```python
from build123d import *

# Parameters (mm, degrees)
SKETCH4_W                        = 24.1
SKETCH4_H                        = 23.8
BOSS_EXTRUDE2_DEPTH              = 2
SKETCH1_W                        = 28.1
SKETCH1_H                        = 28.7
SKETCH1_W_2                      = 24.1
SKETCH1_H_2                      = 23.8
BOSS_EXTRUDE3_DEPTH              = 4
SKETCH6_W                        = 2
SKETCH6_H                        = 2.5
CUT_EXTRUDE2_DEPTH               = 2
SKETCH8_W                        = 7
SKETCH8_H                        = 2
BOSS_EXTRUDE4_DEPTH              = 11.8
SKETCH11_R                       = 6
CUT_EXTRUDE4_DEPTH               = 4
SKETCH12_W                       = 10
SKETCH12_H                       = 2
BOSS_EXTRUDE5_DEPTH              = 7.9
FILLET9_R                        = 5
FILLET10_R                       = 5
SKETCH14_R                       = 2.3
BOSS_EXTRUDE6_DEPTH              = 2.5
DOME3_FACE_RADIUS                = 2.3
DOME3_HEIGHT                     = 1
FILLET11_R                       = 2
FILLET12_R                       = 2
FILLET13_R                       = 2
FILLET14_R                       = 2
BOSS_EXTRUDE7_DEPTH              = 3
SKETCH19_R                       = 0.3
CUT_EXTRUDE6_DEPTH               = 2
CBORE_START                      = -0.2
CBORE_FOR_M1_6_SHCS1_OUTLINE_R   = 1.85
CBORE_FOR_M1_6_SHCS1_DEPTH       = 2.2
CBORE_START_2                    = -3
CBORE_FOR_M1_6_SHCS1_2_OUTLINE_R = 1
CBORE_FOR_M1_6_SHCS1_2_DEPTH     = 2.8
CUT_EXTRUDE8_DEPTH               = 2


# Read off the part's stored shape, not the designer's step: CBORE for M1.6 SHCS1
with BuildPart() as part:
    # Sketch4 → Boss-Extrude2 (new body)
    with BuildSketch(Plane.XY):
        with Locations((14.05, 13.9)):
            Rectangle(SKETCH4_W, SKETCH4_H)
    extrude(amount=BOSS_EXTRUDE2_DEPTH)

    # Sketch1 → Boss-Extrude3 (add)
    with BuildSketch(Plane.XY):
        with Locations((14.05, 14.35)):
            Rectangle(SKETCH1_W, SKETCH1_H)
        with Locations((14.05, 13.9)):
            Rectangle(SKETCH1_W_2, SKETCH1_H_2, mode=Mode.SUBTRACT)
    extrude(amount=BOSS_EXTRUDE3_DEPTH)

    # Sketch6 → Cut-Extrude2 (cut)
    with BuildSketch(Plane.XY.offset(4)):
        with Locations((1, 19.15)):
            Rectangle(SKETCH6_W, SKETCH6_H)
        with Locations((27.1, 19.15)):
            Rectangle(SKETCH6_W, SKETCH6_H)
    extrude(amount=-CUT_EXTRUDE2_DEPTH, mode=Mode.SUBTRACT)

    # Sketch8 → Boss-Extrude4 (add)
    with BuildSketch(Plane.XY):
        with Locations((-1.5, 21.4)):
            Rectangle(SKETCH8_W, SKETCH8_H)
        with Locations((29.6, 21.4)):
            Rectangle(SKETCH8_W, SKETCH8_H)
    extrude(amount=BOSS_EXTRUDE4_DEPTH)

    # Sketch11 → Cut-Extrude4 (cut)
    with BuildSketch(Plane(origin=(0, 25.8, 0), x_dir=(-1, 0, 0), z_dir=(0, -1, 0))):
        with Locations((-8, -8)):
            Circle(SKETCH11_R)
    extrude(amount=-CUT_EXTRUDE4_DEPTH, mode=Mode.SUBTRACT)

    # Sketch12 → Boss-Extrude5 (add)
    with BuildSketch(Plane.XY.offset(4)):
        with Locations((7.9, 1)):
            Rectangle(SKETCH12_W, SKETCH12_H)
    extrude(amount=BOSS_EXTRUDE5_DEPTH)

    # Fillet9
    fillet9_edges = [part.edges().sort_by_distance(p)[0] for p in [
        (2.9, 1, 11.9),
    ]]
    fillet(fillet9_edges, radius=FILLET9_R)

    # Fillet10
    fillet10_edges = [part.edges().sort_by_distance(p)[0] for p in [
        (12.9, 1, 11.9),
    ]]
    fillet(fillet10_edges, radius=FILLET10_R - 0.0001)  # a hair under: the kernel refuses the full size

    # Sketch14 → Boss-Extrude6 (add)
    with BuildSketch(Plane(origin=(0, 0, 0), x_dir=(-1, 0, 0), z_dir=(0, -1, 0))):
        with Locations(Location((-7.9, -7.9, 0), (0, 0, 270))):
            Circle(SKETCH14_R)
    extrude(amount=BOSS_EXTRUDE6_DEPTH)

    # Dome3: a dome of height H over a round flat face of radius A is a cap of a sphere of radius (A * A + H * H) / (2 * H)
    dome3_r = (DOME3_FACE_RADIUS * DOME3_FACE_RADIUS + DOME3_HEIGHT * DOME3_HEIGHT) / (2 * DOME3_HEIGHT)
    dome3_base = Plane((7.9, -2.5, 7.9), z_dir=(0, -1, 0))
    with Locations(dome3_base.offset(DOME3_HEIGHT - dome3_r)):
        dome3_ball = Sphere(dome3_r, mode=Mode.PRIVATE)
    add(split(dome3_ball, bisect_by=dome3_base, keep=Keep.TOP, mode=Mode.PRIVATE))

    # Fillet11
    fillet11_edges = [part.edges().sort_by_distance(p)[0] for p in [
        (2, 21.4, 11.8),
    ]]
    fillet(fillet11_edges, radius=FILLET11_R)

    # Fillet12
    fillet12_edges = [part.edges().sort_by_distance(p)[0] for p in [
        (-5, 21.4, 11.8),
    ]]
    fillet(fillet12_edges, radius=FILLET12_R)

    # Fillet13
    fillet13_edges = [part.edges().sort_by_distance(p)[0] for p in [
        (33.1, 21.4, 11.8),
    ]]
    fillet(fillet13_edges, radius=FILLET13_R)

    # Fillet14
    fillet14_edges = [part.edges().sort_by_distance(p)[0] for p in [
        (26.1, 21.4, 11.8),
    ]]
    fillet(fillet14_edges, radius=FILLET14_R)

    # Sketch16 → Boss-Extrude7 (add)
    with BuildSketch(Plane.XY):
        Polygon((33.1, 22.4), (28.1, 22.4), (28.1, 28.7), (0, 28.7), (0, 22.4), (-5, 22.4), (-5, 20.4), (0, 20.4), (0, 0), (28.1, 0), (28.1, 20.4), (33.1, 20.4), align=None)
    extrude(amount=-BOSS_EXTRUDE7_DEPTH)

    # Sketch19 → Cut-Extrude6 (cut)
    with BuildSketch(Plane.XY):
        with Locations((19.57, 15.62440581)):
            Circle(SKETCH19_R)
        with Locations((13.25, 22.33440581)):
            Circle(SKETCH19_R)
        with Locations(Location((6.93, 15.62440581, 0), (0, 0, 180))):
            Circle(SKETCH19_R)
        with Locations(Location((13.25, 8.91440581, 0), (0, 0, 180))):
            Circle(SKETCH19_R)
    extrude(amount=CUT_EXTRUDE6_DEPTH, mode=Mode.SUBTRACT)

    # CBORE for M1.6 SHCS1 outline → CBORE for M1.6 SHCS1 (cut)
    with BuildSketch(Plane.XY.offset(CBORE_START)):
        with Locations((14.05, 8.91440581)):
            Circle(CBORE_FOR_M1_6_SHCS1_OUTLINE_R)
        with Locations((19.57, 16.4)):
            Circle(CBORE_FOR_M1_6_SHCS1_OUTLINE_R)
        with Locations((14.05, 22.33440581)):
            Circle(CBORE_FOR_M1_6_SHCS1_OUTLINE_R)
        with Locations((6.93, 16.4)):
            Circle(CBORE_FOR_M1_6_SHCS1_OUTLINE_R)
    extrude(amount=CBORE_FOR_M1_6_SHCS1_DEPTH, mode=Mode.SUBTRACT)

    # CBORE for M1.6 SHCS1 2 outline → CBORE for M1.6 SHCS1 2 (cut)
    with BuildSketch(Plane.XY.offset(CBORE_START_2)):
        with Locations((14.05, 8.91440581)):
            Circle(CBORE_FOR_M1_6_SHCS1_2_OUTLINE_R)
        with Locations((19.57, 16.4)):
            Circle(CBORE_FOR_M1_6_SHCS1_2_OUTLINE_R)
        with Locations((14.05, 22.33440581)):
            Circle(CBORE_FOR_M1_6_SHCS1_2_OUTLINE_R)
        with Locations((6.93, 16.4)):
            Circle(CBORE_FOR_M1_6_SHCS1_2_OUTLINE_R)
    extrude(amount=CBORE_FOR_M1_6_SHCS1_2_DEPTH, mode=Mode.SUBTRACT)

    # Sketch10 → Cut-Extrude8 (cut)
    with BuildSketch(Plane(origin=(0, 20.4, 0), x_dir=(-1, 0, 0), z_dir=(0, -1, 0))):
        with BuildLine():
            Line((-29.35, -6.65), (-28.35, -6.65))
            ThreePointArc((-28.35, -6.65), (-27.1, -7.9), (-28.35, -9.15))
            Line((-28.35, -9.15), (-29.35, -9.15))
            ThreePointArc((-29.35, -9.15), (-30.6, -7.9), (-29.35, -6.65))
        make_face()
        with BuildLine():
            Line((1.25, -6.65), (0.25, -6.65))
            ThreePointArc((0.25, -6.65), (-1, -7.9), (0.25, -9.15))
            Line((0.25, -9.15), (1.25, -9.15))
            ThreePointArc((1.25, -9.15), (2.5, -7.9), (1.25, -6.65))
        make_face()
    extrude(amount=-CUT_EXTRUDE8_DEPTH, mode=Mode.SUBTRACT)


solid = part.part
```
Verification items for the finished model (mm, model axes). A direction names the side the tool comes from. Round coordinates to 2 decimals unless told otherwise and drop trailing zeros. Write each loop counter-clockwise with the first axis right and the second up, starting at its lowest first coordinate (ties: lowest second). Pieces come first, ordered by that corner, then holes.
1. Access from +Z, -Z, +X, -X, +Y, -Y to the whole of each face (thin tool, end or side, straight path). Record for faces 1 (the flat face through (-1, 21, 9.15)), 2 (the flat face through (20, 27, 4)), 3 (the cylindrical face through (15.004, 22.635, -1.62)), 4 (the flat face through (20.4, 15.6, -0.2)).
2. Section check B-B on z = 11.25. Enter the section's corners in (x, y), plus the area to 3 significant figures.
3. Section check C-C on x = 19.57. Enter the section's corners in (y, z), plus the area to 3 significant figures.
4. Section check A-A on y = 16.4. Enter the section's corners in (x, z).
5. Section check D-D on x = 14.05. Enter the section's corners in (y, z), plus the area to 3 significant figures.
6. Draft check along Z on faces 5 (the cylindrical face through (27.1, 21.4, 7.9)), 6 (the cylindrical face through (10.145, -1.232, 7.401)), 7 (the flat face through (1, 26, 4)), 8 (the flat face through (29, 21, 9.15)). Enter one of: +Z half, -Z half, draft (parallel to the pull), parting line (faces both ways), or undercut.
7. Scan lines: L1, parallel to Y at x = 14.05, z = -2.35; L2, parallel to Y at x = 14.05, z = 1.15; L3, parallel to X at y = 5, z = 3. Record each from-to range of solid material in increasing order.
8. Gauge pin test, flat ends, axial feed: P1, Ø10, axis at x = 18.5, y = 17, coming from the +Z side; P2, Ø5, axis at x = 20.5, y = 25.5, coming from the +Z side; P3, Ø6, axis at x = 19.57, y = 16.4, coming from the -Z side; P4, Ø6, axis at x = 27.5, y = 24.5, coming from the +Z side. Record the tip position at first contact, or that the pin passes through.
Answer:
1. face 1: +Y, -Y
1. face 2: +Z, +X, -X, +Y
1. face 3: +Z, -Z
1. face 4: +Z
2. outline: (-4.38, 20.4) - (1.38, 20.4) - (1.38, 22.4) - (-4.38, 22.4) - close; (5.43, 0) - (10.37, 0) - (10.37, 2) - (5.43, 2) - close; (26.72, 20.4) - (32.48, 20.4) - (32.48, 22.4) - (26.72, 22.4) - close
2. area: 32.9 mm2
3. outline: (0, -3) - (15.4, -3) - (15.4, -0.2) - (14.55, -0.2) - (14.55, 2) - (2, 2) - (2, 4) - (0, 4) - close; (17.4, -3) - (28.7, -3) - (28.7, 4) - (25.8, 4) - (25.8, 2) - (18.25, 2) - (18.25, -0.2) - (17.4, -0.2) - close
3. area: 140 mm2
4. outline: (0, -3) - (5.93, -3) - (5.93, -0.2) - (5.08, -0.2) - (5.08, 2) - (2, 2) - (2, 4) - (0, 4) - close; (7.93, -3) - (18.57, -3) - (18.57, -0.2) - (17.72, -0.2) - (17.72, 2) - (8.78, 2) - (8.78, -0.2) - (7.93, -0.2) - close; (20.57, -3) - (28.1, -3) - (28.1, 4) - (26.1, 4) - (26.1, 2) - (21.42, 2) - (21.42, -0.2) - (20.57, -0.2) - close
5. outline: (0, -3) - (7.91, -3) - (7.91, -0.2) - (7.06, -0.2) - (7.06, 2) - (2, 2) - (2, 4) - (0, 4) - close; (9.91, -3) - (21.33, -3) - (21.33, -0.2) - (20.48, -0.2) - (20.48, 2) - (10.76, 2) - (10.76, -0.2) - (9.91, -0.2) - close; (23.33, -3) - (28.7, -3) - (28.7, 4) - (25.8, 4) - (25.8, 2) - (24.18, 2) - (24.18, -0.2) - (23.33, -0.2) - close
5. area: 126 mm2
6. face 5: undercut
6. face 6: parting line
6. face 7: +Z half
6. face 8: undercut
7. L1: y = 0 to 7.91, 9.91 to 21.33, 23.33 to 28.7
7. L2: y = 0 to 7.06, 10.76 to 20.48, 24.18 to 28.7
7. L3: x = 0 to 2, 26.1 to 28.1
8. P1: stops at z = 2
8. P2: stops at z = 4
8. P3: stops at z = -3
8. P4: stops at z = 11.8
